Work out the finished part from the listing and answer in its coordinate system (mm). A direction names the side the tool comes from. Coordinates: 2 decimals unless noted, no trailing zeros. Write each question's results on one line, items separated by ' | '. Start each with the question number.
1. Determine the mould class of faces 4 (the cylindrical face through (18.69, -15.7, 5)), 5 (the flat face through (20, -4.283, 6)), 6 (the flat face through (0, 6, 0)) for opening direction Z: released by +Z, released by -Z, zero draft, split by the parting line, or undercut.
2. A cutting plane is placed at A-A on z = 3. State how many separate pieces and enclosed holes the cut face has, then the cut area to 3 significant figures.
3. Find the intervals of material crossed by line 1 along Z through (x, y) = (-20, -13.5); line 2 along Y through (x, z) = (-16.5, 8); line 3 along Y through (x, z) = (-8, 5.5), in increasing order. Write a range as [from, to].
4. Which of the six approach directions +Z, -Z, +X, -X, +Y, -Y give full straight-line access (tool end or side, diameter ignored) to faces 1 (the flat face through (0, 6, 12)), 2 (the cylindrical face through (-21.31, -15.7, 5)), 3 (the flat face through (24.5, -8, 6))?
5. Each of these flat-tipped pins is pushed along its axis until it touches: P1, Ø2.5, axis at x = 20, z = 6, coming from the +Y side; P2, Ø2, axis at x = -20, z = 6, coming from the +Y side; P3, Ø4.5, axis at x = -20.5, z = 7.5, coming from the +Y side. Where does it stop, or does it pass through?
from build123d import *

# Parameters (mm, degrees)
SKETCH1_W           = 64
SKETCH1_H           = 40
BOSS_EXTRUDE1_DEPTH = 12
CUT_EXTRUDE1_DEPTH  = 13.0000001
SKETCH3_R           = 1.65
CUT_EXTRUDE4_DEPTH  = 10
SKETCH5_W           = 9
SKETCH5_H           = 7
CUT_EXTRUDE5_DEPTH  = 13.0000001


with BuildPart() as part:
    # Sketch1 → Boss-Extrude1 (new body)
    with BuildSketch(Plane.XY):
        with BuildLine():
            Line((-32, 55), (-32, 20))
            Line((-32, 20), (21.894736842, 20))
            add(Edge.make_bspline(
                [(-32, 55), (-25.467258538, 62.875582676), (-5.817351499, 72.029269909), (19.334385291, 52.075193803), (23.775907594, 32.709936379), (21.894736842, 20)],
                knots=[0, 0, 0, 0, 0.37053834, 0.573066511, 1, 1, 1, 1], degree=3))
        make_face()
        Rectangle(SKETCH1_W, SKETCH1_H)
    extrude(amount=BOSS_EXTRUDE1_DEPTH)

    # Sketch2 → Cut-Extrude1 (cut, through all)
    with BuildSketch(Plane.XY.offset(12)):
        with BuildLine():
            Line((4.2, 23.284599918), (4.2, 52.5))
            Line((4.2, 52.5), (-20.2, 52.5))
            Line((-20.2, 52.5), (-20.2, 23.284599918))
            ThreePointArc((-20.2, 23.284599918), (-8, 19.4), (4.2, 23.284599918))
        make_face()
        with BuildLine():
            Line((-20.2, 52.5), (4.2, 52.5))
            Line((4.2, 52.5), (4.2, 23.284599918))
            ThreePointArc((4.2, 23.284599918), (10.743398838, 30.81005676), (13.1, 40.5))
            ThreePointArc((13.1, 40.5), (-17.68994324, 59.243398838), (-20.2, 23.284599918))
            Line((-20.2, 23.284599918), (-20.2, 52.5))
        make_face()
    extrude(amount=-CUT_EXTRUDE1_DEPTH, mode=Mode.SUBTRACT)

    # Sketch3 → Cut-Extrude4 (cut)
    with BuildSketch(Plane.XZ.offset(20)):
        with Locations((-20, 6)):
            Circle(SKETCH3_R)
        with Locations((20, 6)):
            Circle(SKETCH3_R)
    extrude(amount=-CUT_EXTRUDE4_DEPTH, mode=Mode.SUBTRACT)

    # Sketch5 → Cut-Extrude5 (cut, through all)
    with BuildSketch(Plane.XY.offset(12)):
        with Locations((-20, -7.782850087)):
            Rectangle(SKETCH5_W, SKETCH5_H)
        with Locations((20, -7.782850087)):
            Rectangle(SKETCH5_W, SKETCH5_H)
    extrude(amount=-CUT_EXTRUDE5_DEPTH, mode=Mode.SUBTRACT)


solid = part.part
Values:
1) face 4: undercut | face 5: zero draft | face 6: released by -Z
2) separate pieces: 1 | enclosed holes: 3 | area: 3,220 mm^2
3) line 1: [0, 4.35], [7.65, 12] | line 2: [-20, -11.28], [-4.28, 21.19], [59.81, 65.28] | line 3: [-20, 19.4], [61.6, 66.76]
4) face 1: +Z, +X, -X, +Y, -Y | face 2: -Y | face 3: +Z, -Z
5) P1: y = 45.6 | P2: y = 64.36 | P3: y = 64.66
